The listing builds one solid part. Answer for the finished solid, in the listing's coordinates (mm). Face numbers are marked on the shaded views. A direction names the side the tool comes from. Round coordinates to 2 decimals unless told otherwise and drop trailing zeros. Write each loop counter-clockwise with the first axis right and the second up, starting at its lowest first coordinate (ties: lowest second). Pieces come first, ordered by that corner, then holes. Notation, with made-up numbers: (49.25, -25) - (101.25, -25) arc R27 cw to (101.25, -8) - close; hole circle Ø11 at (22, -7). An arc over 180 degrees is marked (long way). Return JSON: item names as keys, results as strings. Group by question number.
(1) Section B-B, the plane y = 0 is taken. Write down the section's boundary in (x, z).
(2) Which of the six approach directions +Z, -Z, +X, -X, +Y, -Y give full straight-line access (tool end or side, diameter ignored) to the marked faces 4, 5, 6 and 7?
(3) Find the intervals of material crossed by line 1 along Y through (x, z) = (0, -21.5); line 2 along X through (y, z) = (0.5, -5.5); line 3 along Z through (x, y) = (10, -10), in increasing order. Write a range as [from, to].
(4) Section A-A, the plane z = -14.75 is taken. Write down the section's boundary in (x, y), then the cut area to 3 significant figures.
(5) Determine the mould class of the marked faces 1, 2 and 3 for opening direction Y: +Y half, -Y half, draft (parallel to the pull), parting line (faces both ways), or undercut.
(6) Each of these flat-tipped pins is pushed along its axis until it touches: pin 1 (2 mm diameter, centred on x = 3.5, z = -7.5, fed in from +Y); pin 2 (4.5 mm diameter, centred on x = 0.5, y = -11.5, fed in from -Z); pin 3 (1 mm diameter, centred on x = -7, z = -6, fed in from +Y). Where does it stop, or does it pass through?
(7) Section D-D, the plane z = -20.5 is taken. Write down the section's boundary in (x, y), then the cut area to 3 significant figures.
```python
from build123d import *

# Parameters (mm, degrees)
TAGLIO_ESTRUSIONE1_DEPTH = 35.18332927
SCHIZZO3_W               = 16.3
SCHIZZO3_H               = 2
FORO_4_0_4_1_D           = 4.00000006
FORO_4_0_4_1_DEPTH       = 8


with BuildPart() as part:
    # Schizzo1 → Rivoluzione1 (revolve)
    with BuildSketch(Plane.XZ, mode=Mode.PRIVATE) as rivoluzione1_sk:
        Polygon((16, -3.5), (0, -3.5), (0, -25.5), (18.5, -25.5), (18.5, -16.5), (16, -14), align=None)
    revolve(rivoluzione1_sk.sketch.rotate(Axis((0, 0, -3.5), (0, 0, -1)), 180), axis=Axis((0, 0, -3.5), (0, 0, -1)))

    # Schizzo2 → Taglio-Estrusione1 (cut, through all)
    with BuildSketch(Plane(origin=(0, 0, -25.5), x_dir=(-1, 0, 0), z_dir=(0, 0, -1))):
        with BuildLine():
            Line((8.4, -6.131883887), (8.4, 6.131883887))
            ThreePointArc((8.4, 6.131883887), (7.353910524, 7.353910524), (6.131883887, 8.4))
            Line((6.131883887, 8.4), (-6.131883887, 8.4))
            ThreePointArc((-6.131883887, 8.4), (-7.353910524, 7.353910524), (-8.4, 6.131883887))
            Line((-8.4, 6.131883887), (-8.4, -6.131883887))
            ThreePointArc((-8.4, -6.131883887), (-7.353910524, -7.353910524), (-6.131883887, -8.4))
            Line((-6.131883887, -8.4), (6.131883887, -8.4))
            ThreePointArc((6.131883887, -8.4), (7.353910524, -7.353910524), (8.4, -6.131883887))
        make_face()
    extrude(amount=-TAGLIO_ESTRUSIONE1_DEPTH, mode=Mode.SUBTRACT)

    # Schizzo3 → Taglia-Rivoluzione1 (revolve, cut)
    with BuildSketch(Plane(origin=(0, 0, 0), x_dir=(1, 0, 0), z_dir=(0, 1, 0))):
        with Locations((8.15, 24.5)):
            Rectangle(SCHIZZO3_W, SCHIZZO3_H)
    revolve(axis=Axis((0, 0, -25.5), (0, 0, 1)), mode=Mode.SUBTRACT)

    # Foro Ø4.0 (4)-1
    with Locations(Plane(origin=(0, 0, -23.5), x_dir=(-1, 0, 0), z_dir=(0, 0, -1))):
        with Locations((-12, 0), (0, -12), (12, 0), (0, 12)):
            Hole(FORO_4_0_4_1_D / 2, depth=FORO_4_0_4_1_DEPTH)


solid = part.part
```
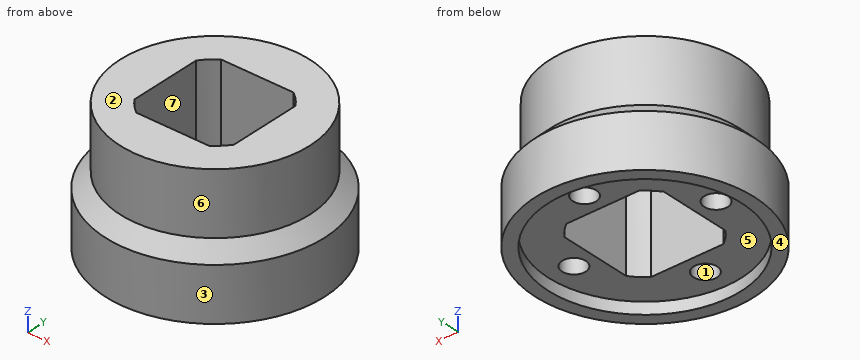
Working result:
{
 "1": {"outline": "(-18.5, -25.5) - (-16.3, -25.5) - (-16.3, -23.5) - (-14, -23.5) - (-14, -15.5) - (-10, -15.5) - (-10, -23.5) - (-8.4, -23.5) - (-8.4, -3.5) - (-16, -3.5) - (-16, -14) - (-18.5, -16.5) - close; (8.4, -23.5) - (10, -23.5) - (10, -15.5) - (14, -15.5) - (14, -23.5) - (16.3, -23.5) - (16.3, -25.5) - (18.5, -25.5) - (18.5, -16.5) - (16, -14) - (16, -3.5) - (8.4, -3.5) - close"},
 "2": {"face 4": "-Z, +X, -X, +Y, -Y", "face 5": "-Z", "face 6": "+Z", "face 7": "+Z, -Z"},
 "3": {"line 1": "y = [-18.5, -14], [-10, -8.4], [8.4, 10], [14, 18.5]", "line 2": "x = [-15.99, -8.4], [8.4, 15.99]", "line 3": "z = [-23.5, -3.5]"},
 "4": {"outline": "circle Ø33.5 at (0, 0); hole (-8.4, -6.13) arc R10.4 ccw to (-6.13, -8.4) - (6.13, -8.4) arc R10.4 ccw to (8.4, -6.13) - (8.4, 6.13) arc R10.4 ccw to (6.13, 8.4) - (-6.13, 8.4) arc R10.4 ccw to (-8.4, 6.13) - close", "area": "608 mm^2"},
 "5": {"face 1": "undercut", "face 2": "draft", "face 3": "parting line"},
 "6": {"pin 1": "stops at y = 15.8", "pin 2": "stops at z = -23.5", "pin 3": "stops at y = 14.62"},
 "7": {"outline": "circle Ø37 at (0, 0); hole circle Ø4 at (-12, 0); hole (-8.4, -6.13) arc R10.4 ccw to (-6.13, -8.4) - (6.13, -8.4) arc R10.4 ccw to (8.4, -6.13) - (8.4, 6.13) arc R10.4 ccw to (6.13, 8.4) - (-6.13, 8.4) arc R10.4 ccw to (-8.4, 6.13) - close; hole circle Ø4 at (0, -12); hole circle Ø4 at (0, 12); hole circle Ø4 at (12, 0)", "area": "752 mm^2"}
}
